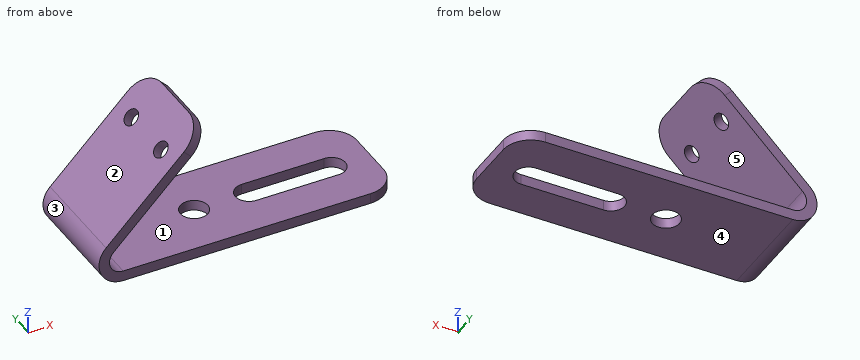
```python
from build123d import *

# Parameters (mm, degrees)
F1_DEPTH = 9.525
F2_R     = 2.5
F3_DEPTH = 1.901
F4_R     = 1.5
F5_DEPTH = 10
F6_R     = 5


with BuildPart() as f1:
    # F0 (on Front) → F1 (new body, symmetric)
    with BuildSketch(Plane.XZ):
        with BuildLine():
            Line((14.5663996924, 20.7889393669), (-3.1112698372, 3.1112698372))
            ThreePointArc((-3.1112698372, 3.1112698372), (-4.065069943, -1.6838071024), (0, -4.4))
            Line((0, -4.4), (50, -4.4))
            Line((50, -4.4), (50, -2.5))
            Line((50, -2.5), (0, -2.5))
            ThreePointArc((0, -2.5), (-2.3096988313, -0.9567085809), (-1.767766953, 1.767766953))
            Line((-1.767766953, 1.767766953), (15.9099025767, 19.4454364826))
            Line((15.9099025767, 19.4454364826), (14.5663996924, 20.7889393669))
        make_face()
    extrude(amount=F1_DEPTH, both=True)

    # F2 (on face) → F3 (cut, through all)
    with BuildSketch(Plane.XY.offset(-2.5)):
        with BuildLine():
            Line((43, 2.5), (28, 2.5))
            ThreePointArc((28, 2.5), (25.5, 0), (28, -2.5))
            Line((28, -2.5), (43, -2.5))
            ThreePointArc((43, -2.5), (45.5, 0), (43, 2.5))
        make_face()
        with Locations((18, 0)):
            Circle(F2_R)
    extrude(amount=-F3_DEPTH, mode=Mode.SUBTRACT)

    # F4 (on face) → F5 (cut)
    with BuildSketch(Plane(origin=(-3.1112698372, 0, 3.1112698372), x_dir=(0, -1, 0), z_dir=(-0.7071067812, 0, 0.7071067812))):
        with Locations((-5.025, 17.5)):
            Circle(F4_R)
        with Locations((5.025, 17.5)):
            Circle(F4_R)
    extrude(amount=-F5_DEPTH, mode=Mode.SUBTRACT)

    # F6
    f6_edges = [f1.edges().sort_by_distance(p)[0] for p in [
        (15.238151, 9.525, 20.117188),
        (50, -9.525, -3.45),
        (15.238151, -9.525, 20.117188),
        (50, 9.525, -3.45),
    ]]
    fillet(f6_edges, radius=F6_R)


solid = f1.part
```
Check sheet for the modelled part. Datum: model origin and axes. Units: mm. Face numbers are marked on the shaded views. A direction names the side the tool comes from. Round coordinates to 2 decimals unless told otherwise and drop trailing zeros. Loops run counter-clockwise (first coordinate to the right, second up) from the corner with the lowest first, then second, coordinate; pieces in that order, holes last. Notation, with made-up numbers: (1.25, 75) - (5.25, 75) arc R19 cw to (5.25, 112) - close; hole circle Ø2 at (54.25, -3.75). An arc over 180 degrees is marked (long way). Answer as a JSON object with one key per item and string values. Group by question number.
Q1. Gauge pin test, flat ends, axial feed: P1, Ø3, axis at y = 5, z = 14, coming from the -X side; P2, Ø1, axis at y = 7, z = 3.5, coming from the -X side; P3, Ø2, axis at y = -1.5, z = 6, coming from the -X side. Record the tip position at first contact, or that the pin passes through.
Q2. Sectioned sample at B-B, the plane x = 18. Enter the section's corners in (y, z) (3 decimals), plus the area to 3 significant figures.
Q3. Scan lines: line 1 along Y through (x, z) = (18, -3.6) (3 decimals); line 2 along Z through (x, y) = (28.5, -7.5); line 3 along X through (y, z) = (2.5, -0.25). Record each from-to range of solid material in increasing order. Write a range as [from, to].
Q4. Set-up check for the marked faces 1 and 2: record each of +Z, -Z, +X, -X, +Y, -Y from which the full face is reachable in a straight line by a thin tool's end or side.
Q5. Sectioned sample at C-C, the plane z = 11.5. Enter the section's corners in (x, y) (3 decimals).
Q6. Mould release check, pull along Z, two halves, no side actions. Record for the marked faces 3, 4 and 5: released by +Z, released by -Z, zero draft, split by the parting line, or undercut.
Q7. Sectioned sample at A-A, the plane y = 0. Enter the section's corners in (x, z), plus the area to 3 significant figures.
Solution:
{
 "1": {"P1": "stops at x = 6.28", "P2": "stops at x = -3.22", "P3": "stops at x = -1.22"},
 "2": {"outline": "(-9.525, -4.4) - (-2.5, -4.4) - (-2.5, -2.5) - (-9.525, -2.5) - close; (2.5, -4.4) - (9.525, -4.4) - (9.525, -2.5) - (2.5, -2.5) - close", "area": "26.7 mm²"},
 "3": {"line 1": "y = [-9.525, -2.5], [2.5, 9.525]", "line 2": "z = [-4.4, -2.5]", "line 3": "x = [-4.39, -2.49]"},
 "4": {"face 1": "+X, +Y, -Y", "face 2": "+Z, -X, +Y, -Y"},
 "5": {"outline": "(5.277, -9.525) - (7.964, -9.525) - (7.964, 9.525) - (5.277, 9.525) - close"},
 "6": {"face 3": "split by the parting line", "face 4": "released by -Z", "face 5": "undercut"},
 "7": {"outline": "(-3.11, 3.11) arc R4.4 ccw to (0, -4.4) - (15.5, -4.4) - (15.5, -2.5) - (0, -2.5) arc R2.5 cw to (-1.77, 1.77) - (15.91, 19.45) - (14.57, 20.79) - close; (20.5, -4.4) - (25.5, -4.4) - (25.5, -2.5) - (20.5, -2.5) - close; (45.5, -4.4) - (50, -4.4) - (50, -2.5) - (45.5, -2.5) - close", "area": "110 mm²"}
}
